Geometry: final body of the model. Coordinates: model frame, mm. A direction names the side the tool comes from. Give positions to 0.01 mm unless a question says otherwise; leave off trailing zeros. Write each loop counter-clockwise with the first axis right and the second up, starting at its lowest first coordinate (ties: lowest second). Pieces come first, ordered by that corner, then holes. Notation, with made-up numbers: (77, -5.5) -> (108, -5.5) arc R24 ccw to (108, 10.5) -> close; hole circle Ø5 at (-13, -32.5). An arc over 180 degrees is marked (long way). Answer as a JSON object with one key per item and string values.
from build123d import *

# Parameters (mm, degrees)
F0_R     = 70
F1_DEPTH = 3


# Not quite as in the source:
# - a feature of the source that left no trace in its solid (it failed there, or was rolled back) is left out


with BuildPart() as f1:
    # F0 (on Front) → F1 (new body, symmetric)
    with BuildSketch(Plane.XZ):
        Circle(F0_R)
        Polygon((-30.6363262968, 30.6363262968), (-11.2136737032, 41.85), (11.2136737032, 41.85), (30.6363262968, 30.6363262968), (41.85, 11.2136737032), (41.85, -11.2136737032), (30.6363262968, -30.6363262968), (11.2136737032, -41.85), (-11.2136737032, -41.85), (-30.6363262968, -30.6363262968), (-41.85, -11.2136737032), (-41.85, 11.2136737032), align=None, mode=Mode.SUBTRACT)
    extrude(amount=F1_DEPTH, both=True)


solid = f1.part
Q1. Cut plane C-C (y = 2). Return the cut outline in (x, z).
Values:
{"outline": "circle Ø140 at (0, 0); hole (-41.85, -11.21) -> (-30.64, -30.64) -> (-11.21, -41.85) -> (11.21, -41.85) -> (30.64, -30.64) -> (41.85, -11.21) -> (41.85, 11.21) -> (30.64, 30.64) -> (11.21, 41.85) -> (-11.21, 41.85) -> (-30.64, 30.64) -> (-41.85, 11.21) -> close"}
Q2. Cut plane A-A (x = 0). Return the cut outline in (y, z), and give its area (3 significant figures).
Values:
{"outline": "(-3, -70) -> (3, -70) -> (3, -41.85) -> (-3, -41.85) -> close; (-3, 41.85) -> (3, 41.85) -> (3, 70) -> (-3, 70) -> close", "area": "338 mm²"}
Q3. Cut plane B-B (z = 0). Return the cut outline in (x, y).
Values:
{"outline": "(-70, -3) -> (-41.85, -3) -> (-41.85, 3) -> (-70, 3) -> close; (41.85, -3) -> (70, -3) -> (70, 3) -> (41.85, 3) -> close"}
Q4. Mould query, pull axis X, two halves, no side actions, for faces 1 (the flat face through (-21.061, -0.042, 36.165)), 2 (the cylindrical face through (-55.55, -0.042, -42.594)), 3 (the flat face through (30, 3, 32)). Classes: pulls with the +X half, pulls with the -X half, needs draft (parallel to the pull), parting line crosses it, or undercut.
Values:
{"face 1": "undercut", "face 2": "parting line crosses it", "face 3": "needs draft"}
Q5. Set-up query: faces 4 (the flat face through (36.32, -0.04, -20.79)), 5 (the flat face through (30, -3, 32)). Return all of +Z, -Z, +X, -X, +Y, -Y with unobstructed straight access to the full face (end or side cutting, diameter ignored); none if empty.
Values:
{"face 4": "+Y, -Y", "face 5": "+Z, -Z, +X, -X, -Y"}
Q6. First-contact query: P1, Ø1.8, axis at x = -3, y = -1, coming from the +Z side; P2, Ø3, axis at x = -53.5, y = -1, coming from the -Z side; P3, Ø3, axis at x = -3, y = 0, coming from the -Z side. Flat tips, straight axial feed; report the tip coordinate or a pass-through.
Values:
{"P1": "z = 69.97", "P2": "z = -46.86", "P3": "z = -69.98"}
Q7. Material intervals for L1, parallel to Z at x = 1.5, y = -2.3; L2, parallel to Z at x = 16, y = -0.3; L3, parallel to X at y = -1.25, z = -25, sorted ascending. Write a range as from..to.
Values:
{"L1": "-69.98..-41.85, 41.85..69.98", "L2": "-68.15..-39.09, 39.09..68.15", "L3": "-65.38..-33.89, 33.89..65.38"}
